Geometry: final body of the model. Coordinates: model frame, mm. Face numbers are marked on the shaded views. A direction names the side the tool comes from. Coordinates: 2 decimals unless noted, no trailing zeros. Loops run counter-clockwise (first coordinate to the right, second up) from the corner with the lowest first, then second, coordinate; pieces in that order, holes last. Notation, with made-up numbers: (47.5, 28.25) - (67.5, 28.25) arc R21 ccw to (67.5, 51.25) - close; hole circle Ø8 at (-30.5, 73.5). An arc over 180 degrees is marked (long way). Return JSON: item names as keys, results as strings.
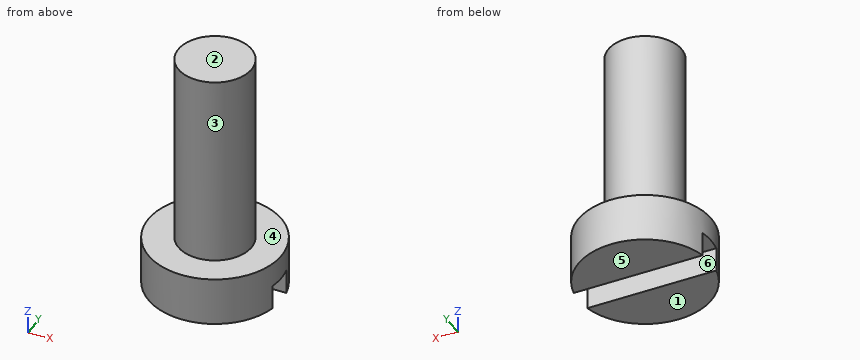
from build123d import *

# Parameters (mm, degrees)
SKETCH1_R          = 2.725
EXTRUDE1_DEPTH     = 2
CUT_EXTRUDE1_DEPTH = 1
SKETCH3_R          = 1.5
EXTRUDE2_DEPTH     = 8


with BuildPart() as part:
    # Sketch1 → Extrude1 (new body)
    with BuildSketch(Plane.XY):
        Circle(SKETCH1_R)
    extrude(amount=EXTRUDE1_DEPTH)

    # Sketch2 → Cut-Extrude1 (cut)
    with BuildSketch(Plane(origin=(0, 0, 0), x_dir=(-1, 0, 0), z_dir=(0, 0, -1))):
        Polygon((3.449801909, 0), (3.449801909, 0.55), (-3.901269584, 0.55), (-3.901269584, -0.55), (3.449801909, -0.55), align=None)
    extrude(amount=-CUT_EXTRUDE1_DEPTH, mode=Mode.SUBTRACT)

    # Sketch3 → Extrude2 (add)
    with BuildSketch(Plane.XY.offset(2)):
        Circle(SKETCH3_R)
    extrude(amount=EXTRUDE2_DEPTH)


solid = part.part
Item 1: Mould query, pull axis Z, two halves, no side actions, for the marked faces 1, 2 and 3. Classes: +Z half, -Z half, draft (parallel to the pull), parting line (faces both ways), or undercut.
Worked out:
{"face 1": "-Z half", "face 2": "+Z half", "face 3": "draft"}
Item 2: Section query D-D, the plane x = 1.8. Return loops of the section in (y, z), and give its area (3 significant figures).
Worked out:
{"outline": "(-2.05, 0) - (-0.55, 0) - (-0.55, 1) - (0.55, 1) - (0.55, 0) - (2.05, 0) - (2.05, 2) - (-2.05, 2) - close", "area": "7.08 mm^2"}
Item 3: Reachability of the marked faces 4, 5 and 6 from +Z, -Z, +X, -X, +Y, -Y: full face, straight path, thin tool, end or side. Return the list, or none.
Worked out:
{"face 4": "+Z", "face 5": "-Z, +X, -X, +Y, -Y", "face 6": "-Z, +X, -X"}
Item 4: Section query A-A, the plane x = 0. Return loops of the section in (y, z) (3 decimals), and give its area (3 significant figures).
Worked out:
{"outline": "(-2.725, 0) - (-0.55, 0) - (-0.55, 1) - (0.55, 1) - (0.55, 0) - (2.725, 0) - (2.725, 2) - (1.5, 2) - (1.5, 10) - (-1.5, 10) - (-1.5, 2) - (-2.725, 2) - close", "area": "33.8 mm^2"}
Item 5: Section query B-B, the plane y = 0. Return loops of the section in (x, z) (3 decimals), and give its area (4 significant figures).
Worked out:
{"outline": "(-2.725, 1) - (2.725, 1) - (2.725, 2) - (1.5, 2) - (1.5, 10) - (-1.5, 10) - (-1.5, 2) - (-2.725, 2) - close", "area": "29.45 mm^2"}
Item 6: Section query C-C, the plane z = 7.5. Return loops of the section in (x, y).
Worked out:
{"outline": "circle Ø3 at (0, 0)"}
Item 7: Ray query, probe 1 along Z at (x, y) = (-1, -1.6); probe 2 along X at (y, z) = (-0.1, 2.75). Return the intervals inside material, ascending. Write a range as from..to.
Worked out:
{"probe 1": "0..2", "probe 2": "-1.5..1.5"}
Item 8: First-contact query: pin 1 Ø3 at (x, z) = (2, 3) entering from +Y; pin 2 Ø3 at (y, z) = (2, 3) entering from +X. Flat tips, straight axial feed; report the tip coordinate or a pass-through.
Worked out:
{"pin 1": "y = 2.58", "pin 2": "x = 2.58"}
